Input: part model. Units: mm. Frame: model coordinates. A direction names the side the tool comes from. Give positions to 0.01 mm unless a question says otherwise; leave off trailing zeros. Order: outer loops, then holes, each group sorted by start corner. A loop starts at its lowest first (then second) coordinate and runs counter-clockwise, first axis right, second up. Notation, with made-up numbers: (30, 38.5) - (52, 38.5) arc R22 ccw to (52, 67.5) - close; hole circle Ø2 at (-4.5, -37). An arc over 180 degrees is marked (long way). Answer in a Markdown table with one row per item. Add a question column.
1. Section query A-A on z = -25. Return loops of the section in (x, y), and give its area (3 significant figures).
2. Section query D-D on y = 11.25. Return loops of the section in (x, z).
3. Contact query for flat-ended pins moving along their axis: pin 1 (3.5 mm diameter, centred on x = 10.2, z = 25, fed in from +Y); pin 2 (4 mm diameter, centred on x = 10.5, z = -31.5, fed in from +Y). Output: stop coordinate, or through.
4. Access query for faces 4 (the face through (1.232, 9.701, -40.646)), 5 (the face through (2.5, 11, 1)). Directions: +Z, -Z, +X, -X, +Y, -Y. A direction counts if a zero-diameter tool reaches every point of the face in a straight line with its end or side. Return the directions, or none.
5. Ray query, line 1 (Y direction, x = 0.85, z = 36.65) (3 decimals); line 2 (Z direction, x = 9, y = 2.25); line 3 (Y direction, x = 7.5, z = -45). Return the intervals inside material, ascending. Write a range as [from, to].
6. Section query C-C on z = 36.65. Return loops of the section in (x, y) (3 decimals).
7. Mould query, pull axis Y, two halves, no side actions, for faces 1 (the face through (1, 19.05, 1)), 2 (the face through (5, 2, -50)), 3 (the face through (1.2, 12.9, 38.8)). Classes: released by +Y, released by -Y, zero draft, split by the parting line, or undercut.
8. Section query B-B on x = 10.2. Return loops of the section in (y, z), and give its area (3 significant figures).
```python
from build123d import *

# Parameters (mm, degrees)
EXTRUDE_THIN1_DEPTH = 50
CUT_EXTRUDE2_REACH  = 58.796
SKETCH4_R           = 4
SKETCH5_R           = 3
CUT_EXTRUDE3_DEPTH  = 57.796170646


with BuildPart() as part:
    # Sketch1 → Extrude-Thin1 (new, symmetric)
    with BuildSketch(Plane.XY):
        Polygon((19.05, 0), (0, 0), (0, 19.05), (2.5, 19.05), (2.5, 2.5), (19.05, 2.5), align=None)
    extrude(amount=EXTRUDE_THIN1_DEPTH, both=True)

    # Sketch4 → Cut-Extrude2 (cut, up to next)
    with BuildSketch(Plane.ZY, mode=Mode.PRIVATE) as cut_extrude2_sk1:
        with Locations((-36.65, 9.525)):
            Circle(SKETCH4_R)
    cut_extrude2_tool1 = extrude(cut_extrude2_sk1.sketch, amount=-CUT_EXTRUDE2_REACH, mode=Mode.PRIVATE) & part.part
    # Sketch4 → Cut-Extrude2 (cut, up to next)
    with BuildSketch(Plane.ZY, mode=Mode.PRIVATE) as cut_extrude2_sk2:
        with Locations((36.65, 9.525)):
            Circle(SKETCH4_R)
    cut_extrude2_tool2 = extrude(cut_extrude2_sk2.sketch, amount=-CUT_EXTRUDE2_REACH, mode=Mode.PRIVATE) & part.part
    add(cut_extrude2_tool1.solids().sort_by_distance((0, 9.525, -36.65))[0], mode=Mode.SUBTRACT)
    add(cut_extrude2_tool2.solids().sort_by_distance((0, 9.525, 36.65))[0], mode=Mode.SUBTRACT)

    # Sketch5 → Cut-Extrude3 (cut, through all)
    with BuildSketch(Plane.XZ):
        with Locations(Location((10.2, 25, 0), (0, 0, 270))):
            Circle(SKETCH5_R)
        with Locations(Location((10.2, -25, 0), (0, 0, 270))):
            Circle(SKETCH5_R)
    extrude(amount=-CUT_EXTRUDE3_DEPTH, mode=Mode.SUBTRACT)


solid = part.part
```
Answer:
| question | item | result |
|---|---|---|
| 1 | outline | (0, 0) - (7.2, 0) - (7.2, 2.5) - (2.5, 2.5) - (2.5, 19.05) - (0, 19.05) - close; (13.2, 0) - (19.05, 0) - (19.05, 2.5) - (13.2, 2.5) - close |
| 1 | area | 74.0 mm² |
| 2 | outline | (0, -50) - (2.5, -50) - (2.5, -40.26) - (0, -40.26) - close; (0, -33.04) - (2.5, -33.04) - (2.5, 33.04) - (0, 33.04) - close; (0, 40.26) - (2.5, 40.26) - (2.5, 50) - (0, 50) - close |
| 3 | pin 1 | passes through |
| 3 | pin 2 | stops at y = 2.5 |
| 4 | face 4 | +X, -X |
| 4 | face 5 | +Z, -Z, +X, +Y |
| 5 | line 1 | y = [0, 5.525], [13.525, 19.05] |
| 5 | line 2 | z = [-50, -27.75], [-22.25, 22.25], [27.75, 50] |
| 5 | line 3 | y = [0, 2.5] |
| 6 | outline | (0, 0) - (19.05, 0) - (19.05, 2.5) - (2.5, 2.5) - (2.5, 5.525) - (0, 5.525) - close; (0, 13.525) - (2.5, 13.525) - (2.5, 19.05) - (0, 19.05) - close |
| 7 | face 1 | released by +Y |
| 7 | face 2 | zero draft |
| 7 | face 3 | undercut |
| 8 | outline | (0, -50) - (2.5, -50) - (2.5, -28) - (0, -28) - close; (0, -22) - (2.5, -22) - (2.5, 22) - (0, 22) - close; (0, 28) - (2.5, 28) - (2.5, 50) - (0, 50) - close |
| 8 | area | 220 mm² |
